from build123d import *

# Parameters (mm, degrees)
SKETCH1_W                         = 71
SKETCH1_H                         = 54
BOSS_EXTRUDE1_DEPTH               = 2.5
M1_4X0_3_TAPPED_HOLE1_D           = 1.1
M1_4X0_3_TAPPED_HOLE1_CSINK_D     = 1.45
M1_4X0_3_TAPPED_HOLE1_CSINK_ANGLE = 90
CUT_EXTRUDE1_DEPTH                = 1.8
SKETCH5_R                         = 6
SKETCH5_R_2                       = 5
SKETCH5_R_3                       = 5.5
CUT_EXTRUDE2_DEPTH                = 1.5
FILLET1_R                         = 2
FILLET2_R                         = 1
SKETCH6_R                         = 1
CUT_EXTRUDE4_DEPTH                = 0.5


with BuildPart() as part:
    # Sketch1 → Boss-Extrude1 (new body)
    with BuildSketch(Plane(origin=(0, 0, 0), x_dir=(1, 0, 0), z_dir=(0, 1, 0))):
        Rectangle(SKETCH1_W, SKETCH1_H)
    extrude(amount=BOSS_EXTRUDE1_DEPTH)

    # M1.4x0.3 Tapped Hole1 (through all)
    with Locations(Plane(origin=(0, 2.5, 0), x_dir=(1, 0, 0), z_dir=(0, 1, 0))):
        with Locations((-33.2, 24.7), (32.5, 24.7), (-33.2, -23), (29.4, -19.4)):
            CounterSinkHole(M1_4X0_3_TAPPED_HOLE1_D / 2, M1_4X0_3_TAPPED_HOLE1_CSINK_D / 2, counter_sink_angle=M1_4X0_3_TAPPED_HOLE1_CSINK_ANGLE)

    # Sketch4 → Cut-Extrude1 (cut)
    with BuildSketch(Plane.XZ):
        with BuildLine():
            Line((-7.748076809, 19), (-33.5, 19))
            Line((-33.5, 19), (-33.5, -20))
            Line((-33.5, -20), (-6.5, -20))
            ThreePointArc((-6.5, -20), (33.487208249, 0.799639875), (-7.748076809, 19))
        make_face()
    extrude(amount=-CUT_EXTRUDE1_DEPTH, mode=Mode.SUBTRACT)

    # Sketch5 → Cut-Extrude2 (cut)
    with BuildSketch(Plane(origin=(0, 2.5, 0), x_dir=(1, 0, 0), z_dir=(0, 1, 0))):
        with Locations((-35.5, -27)):
            Circle(SKETCH5_R)
        with Locations((-35.5, 27)):
            Circle(SKETCH5_R_2)
        with Locations((35.5, 27)):
            Circle(SKETCH5_R_3)
        with BuildLine():
            Line((34.5, -1), (35.5, -1))
            Line((35.5, -1), (35.5, -27))
            Line((35.5, -27), (13.5, -27))
            Line((13.5, -27), (13.5, -26))
            ThreePointArc((13.5, -26), (28.644692027, -17.401541303), (34.5, -1))
        make_face()
    extrude(amount=-CUT_EXTRUDE2_DEPTH, mode=Mode.SUBTRACT)

    # Fillet1
    fillet1_edges = [part.edges().sort_by_distance(p)[0] for p in [
        (35.5, 0.5, 27),
        (-35.5, 0.5, 27),
        (-35.5, 0.5, -27),
        (35.5, 0.5, -27),
    ]]
    fillet(fillet1_edges, radius=FILLET1_R)

    # Fillet2
    fillet2_edges = [part.edges().sort_by_distance(p)[0] for p in [
        (-8, 2.5, 27),
        (-35.5, 2.5, -0.5),
        (-0.25, 2.5, -27),
        (35.5, 2.5, -10.25),
        (28.644692027, 2.5, 17.401541303),
        (13.5, 2.5, 26.5),
        (35, 2.5, 1),
        (-31.964466094, 2.5, -23.464466094),
        (-31.257359313, 2.5, 22.757359313),
    ]]
    fillet(fillet2_edges, radius=FILLET2_R)

    # Sketch6 → Cut-Extrude4 (cut)
    with BuildSketch(Plane(origin=(0, 1, 0), x_dir=(1, 0, 0), z_dir=(0, 1, 0))):
        with Locations((-33.2, 24.7)):
            Circle(SKETCH6_R)
        with Locations((32.5, 24.7)):
            Circle(SKETCH6_R)
        with Locations((29.4, -19.4)):
            Circle(SKETCH6_R)
        with Locations((-33.2, -23)):
            Circle(SKETCH6_R)
    extrude(amount=-CUT_EXTRUDE4_DEPTH, mode=Mode.SUBTRACT)


solid = part.part
Input: part model. Units: mm. Frame: model coordinates. A direction names the side the tool comes from. Give positions to 0.01 mm unless a question says otherwise; leave off trailing zeros. Write each loop counter-clockwise with the first axis right and the second up, starting at its lowest first coordinate (ties: lowest second). Pieces come first, ordered by that corner, then holes. Notation, with made-up numbers: (-16.75, -30) -> (12.25, -30) arc R21 cw to (12.25, -25) -> close; hole circle Ø4 at (-27, 80). An arc over 180 degrees is marked (long way). Use one line per item in the form item = value. Start each with the question number.
1) Set-up query: faces 1 (the flat face through (-34, 1, -26)), 2 (the flat face through (34, 1, -24)), 3 (the cylindrical face through (33.5, 0.9, 0)), 4 (the flat face through (-33, 1, 25)), 5 (the flat face through (-32.5, 0.5, 23)). Return all of +Z, -Z, +X, -X, +Y, -Y with unobstructed straight access to the full face (end or side cutting, diameter ignored); none if empty.
2) Ray query, probe 1 along Z at (x, y) = (-33.2, 0.3); probe 2 along Z at (x, y) = (-33.2, 0.7); probe 3 along X at (y, z) = (0.25, 23). Return the intervals inside material, ascending. Write a range as from..to.
3) Section query A-A on x = 8.5. Return the cut outline in (y, z).
4) Pin query (flat end, axial travel): pin 1 (1.8 mm diameter, centred on x = -33.2, z = -24.7, fed in from +Y); pin 2 (5 mm diameter, centred on x = 10.5, z = -4.5, fed in from -Y); pin 3 (2 mm diameter, centred on x = -33.5, z = 23, fed in from +Y); pin 4 (0.9 mm diameter, centred on x = -33.2, z = 23, fed in from -Y). Return the tip coordinate at first contact, or that it passes through.
5) Section query B-B on z = -16.5. Return the cut outline in (x, y), then the cut area to 3 significant figures.
Outcome:
q1.face_1 = -Z, -X, +Y
q1.face_2 = -Z, +X, +Y
q1.face_3 = -Y
q1.face_4 = +Z, -X, +Y
q1.face_5 = +Y
q2.probe_1 = -27..-25.25, -24.15..-20, 19..22.45, 23.55..27
q2.probe_2 = -27..-25.7, -23.7..-20, 19..22, 24..27
q2.probe_3 = -35.5..-33.75, -32.65..-1.3, 18.3..35.5
q3.outline = (0, -27) -> (1.5, -27) arc R1 ccw to (2.5, -26) -> (2.5, 26) arc R1 ccw to (1.5, 27) -> (0, 27) -> (0, 25) -> (1.8, 25) -> (1.8, -25) -> (0, -25) -> close
q4.pin_1 = 0.5
q4.pin_2 = 1.8
q4.pin_3 = 1
q4.pin_4 = through
q5.outline = (-35.5, 0) -> (-33.5, 0) -> (-33.5, 1.8) -> (27.28, 1.8) -> (27.28, 0) -> (35.5, 0) -> (35.5, 1.5) arc R1 ccw to (34.5, 2.5) -> (-34.5, 2.5) arc R1 ccw to (-35.5, 1.5) -> close
q5.area = 67.7 mm^2
